from build123d import *

# Parameters (mm, degrees)
F1_DEPTH = 25.4
F3_DEPTH = 2.54
F4_SIZE  = 1.27


with BuildPart() as f1:
    # F0 (on Top) → F1 (new body)
    with BuildSketch(Plane.XY):
        Polygon((0, 16.505921), (-25.4, 34.960101), (-15.698063, 5.10061), (-41.098063, -13.35357), (-9.701937, -13.35357), (0, -43.213061), (9.701937, -13.35357), (41.098063, -13.35357), (15.698063, 5.10061), (25.4, 34.960101), align=None)
        Polygon((-12.712114, 4.130416), (-20.568633, 28.310294), (0, 13.366308), (20.568633, 28.310294), (12.712114, 4.130416), (33.280747, -10.81357), (7.856519, -10.81357), (0, -34.993448), (-7.856519, -10.81357), (-33.280747, -10.81357), align=None, mode=Mode.SUBTRACT)
    extrude(amount=F1_DEPTH)

    # F2 (on face) → F3 (join)
    with BuildSketch(Plane.XY.offset(25.4)):
        Polygon((18.684012, 6.070804), (30.231367, 41.609907), (0, 19.645533), (-30.231367, 41.609907), (-18.684012, 6.070804), (-48.915379, -15.89357), (-11.547355, -15.89357), (0, -51.432674), (11.547355, -15.89357), (48.915379, -15.89357), align=None)
        Polygon((0, 16.505921), (25.4, 34.960101), (15.698063, 5.10061), (41.098063, -13.35357), (9.701937, -13.35357), (0, -43.213061), (-9.701937, -13.35357), (-41.098063, -13.35357), (-15.698063, 5.10061), (-25.4, 34.960101), align=None, mode=Mode.SUBTRACT)
        Polygon((15.698063, 5.10061), (25.4, 34.960101), (0, 16.505921), (-25.4, 34.960101), (-15.698063, 5.10061), (-41.098063, -13.35357), (-9.701937, -13.35357), (0, -43.213061), (9.701937, -13.35357), (41.098063, -13.35357), align=None)
        Polygon((-33.280747, -10.81357), (-12.712114, 4.130416), (-20.568633, 28.310294), (0, 13.366308), (20.568633, 28.310294), (12.712114, 4.130416), (33.280747, -10.81357), (7.856519, -10.81357), (0, -34.993448), (-7.856519, -10.81357), align=None, mode=Mode.SUBTRACT)
    extrude(amount=F3_DEPTH)

    # F4
    f4_edges = [f1.edges().sort_by_distance(p)[0] for p in [
        (20.549032, 20.030355, 0),
        (12.7, 25.733011, 0),
        (-12.7, 25.733011, 0),
        (-20.549032, 20.030355, 0),
        (-28.398063, -4.12648, 0),
        (-25.4, -13.35357, 0),
        (-4.850968, -28.283316, 0),
        (4.850968, -28.283316, 0),
        (25.4, -13.35357, 0),
        (28.398063, -4.12648, 0),
    ]]
    chamfer(f4_edges, length=F4_SIZE)


solid = f1.part
Design review of the part built by this model. Coordinates are the model's own, in mm. A direction names the side the tool comes from. Round coordinates to 2 decimals unless told otherwise and drop trailing zeros. Order: outer loops, then holes, each group sorted by start corner. A loop starts at its lowest first (then second) coordinate and runs counter-clockwise, first axis right, second up.
1) Consider section C-C (x = 3.5). State the section outline as (y, z) points, plus the area to 3 significant figures.
The answers:
outline: (-40.66, 25.4) - (-32.44, 25.4) - (-32.44, 1.27) - (-28.33, 0) - (-24.22, 0) - (-24.22, 27.94) - (-40.66, 27.94) - close; (15.91, 0) - (17.48, 0) - (19.05, 1.27) - (19.05, 25.4) - (22.19, 25.4) - (22.19, 27.94) - (15.91, 27.94) - close
area: 343 mm2
2) Machinability: for faces 5 (the flat face through (-10.428, 20.943, 13.774)), 6 (the flat face through (-19.881, 20, 0.644)), 7 (the flat face through (20.48, 19.82, 13.17)), 8 (the flat face through (-30, -15.894, 27)), which of the approach directions +Z, -Z, +X, -X, +Y, -Y give a long, thin tool a straight path to every point of the face, cutting with its end or side? Answer none if there is none.
The answers:
face 5: +Z, -Z
face 6: -Z, -X
face 7: -Z, +X
face 8: +Z, -Z, -X, -Y
3) Draft analysis for pull direction X (two halves, no side actions). For faces 1 (the flat face through (-20.617, 20.239, 13.166)), 2 (the flat face through (28.58, -4.26, 13.17)), 3 (the flat face through (-26, -13.354, 13)), 4 (the flat face through (-12.512, 24.822, 0.644)), state which applies: released by +X, released by -X, zero draft, split by the parting line, or undercut.
The answers:
face 1: released by -X
face 2: released by +X
face 3: zero draft
face 4: undercut
4) Clearance check with flat-ended pins moving along their axes: pin 1 Ø5 at (y, z) = (18, 3.5) entering from +X; pin 2 Ø6 at (y, z) = (-24, 13) entering from +X; pin 3 Ø12.5 at (x, z) = (-18.5, 12) entering from +Y; pin 4 Ø5 at (x, y) = (-27, 31) entering from +Z. State where each tip first meets the part, or that it passes through.
The answers:
pin 1: stops at x = 20.7
pin 2: stops at x = 7.22
pin 3: stops at y = 34.49
pin 4: stops at z = 27.94
5) Consider section D-D (y = -40.5). State the section outline as (x, z) points.
The answers:
outline: (-3.55, 25.4) - (-0.88, 25.4) - (-0.88, 1.27) - (0, 0.43) - (0.88, 1.27) - (0.88, 25.4) - (3.55, 25.4) - (3.55, 27.94) - (-3.55, 27.94) - close
6) Consider section B-B (z = 9). State the section outline as (x, y) points, plus the area to 3 significant figures.
The answers:
outline: (-41.1, -13.35) - (-9.7, -13.35) - (0, -43.21) - (9.7, -13.35) - (41.1, -13.35) - (15.7, 5.1) - (25.4, 34.96) - (0, 16.51) - (-25.4, 34.96) - (-15.7, 5.1) - close; hole (-33.28, -10.81) - (-7.86, -10.81) - (0, -34.99) - (7.86, -10.81) - (33.28, -10.81) - (12.71, 4.13) - (20.57, 28.31) - (0, 13.37) - (-20.57, 28.31) - (-12.71, 4.13) - close
area: 722 mm2
7) For L1, parallel to X at y = 23, z = 11.5; L2, parallel to Y at x = -28, z = 13.25; L3, parallel to Y at x = 33, z = 18.5, list the stretches that pass through material, from the lowest coordinate up.
The answers:
L1: x = -21.51 to -18.84, -13.26 to -8.94, 8.94 to 13.26, 18.84 to 21.51
L2: y = -13.35 to -10.81, -6.98 to -3.84
L3: y = -13.35 to -10.81, -10.61 to -7.47
8) Consider section A-A (y = -3). State the section outline as (x, z) points.
The answers:
outline: (-31.17, 25.4) - (-26.85, 25.4) - (-26.85, 1.27) - (-24.69, 0) - (-22.53, 0) - (-22.53, 27.94) - (-31.17, 27.94) - close; (22.53, 0) - (24.69, 0) - (26.85, 1.27) - (26.85, 25.4) - (31.17, 25.4) - (31.17, 27.94) - (22.53, 27.94) - close
